```python
from build123d import *

# Parameters (mm, degrees)
SKETCH_1_W          = 120
SKETCH_1_H          = 19
EXTRUDE_1_DEPTH     = 3
SKETCH_2_R          = 1.5
CUT_EXTRUDE_1_DEPTH = 3


with BuildPart() as part:
    # Эскиз1 → Бобышка-Вытянуть1 (new body)
    with BuildSketch(Plane(origin=(0, 0, 0), x_dir=(1, 0, 0), z_dir=(0, 1, 0))):
        Rectangle(SKETCH_1_W, SKETCH_1_H)
    extrude(amount=EXTRUDE_1_DEPTH)

    # Эскиз2 → Вырез-Вытянуть1 (cut)
    with BuildSketch(Plane(origin=(0, 3, 0), x_dir=(1, 0, 0), z_dir=(0, 1, 0))):
        with Locations((-51.862444671, 3.5)):
            Circle(SKETCH_2_R)
        with Locations((-56.963668737, -3.5)):
            Circle(SKETCH_2_R)
        with Locations((-31.862444671, 3.5)):
            Circle(SKETCH_2_R)
        with Locations((-36.963668737, -3.5)):
            Circle(SKETCH_2_R)
        with Locations((-11.862444671, 3.5)):
            Circle(SKETCH_2_R)
        with Locations((-16.963668737, -3.5)):
            Circle(SKETCH_2_R)
        with Locations((8.137555329, 3.5)):
            Circle(SKETCH_2_R)
        with Locations((3.036331263, -3.5)):
            Circle(SKETCH_2_R)
        with Locations((28.137555329, 3.5)):
            Circle(SKETCH_2_R)
        with Locations((23.036331263, -3.5)):
            Circle(SKETCH_2_R)
        with Locations((48.137555329, 3.5)):
            Circle(SKETCH_2_R)
        with Locations((43.036331263, -3.5)):
            Circle(SKETCH_2_R)
    extrude(amount=-CUT_EXTRUDE_1_DEPTH, mode=Mode.SUBTRACT)


solid = part.part
```
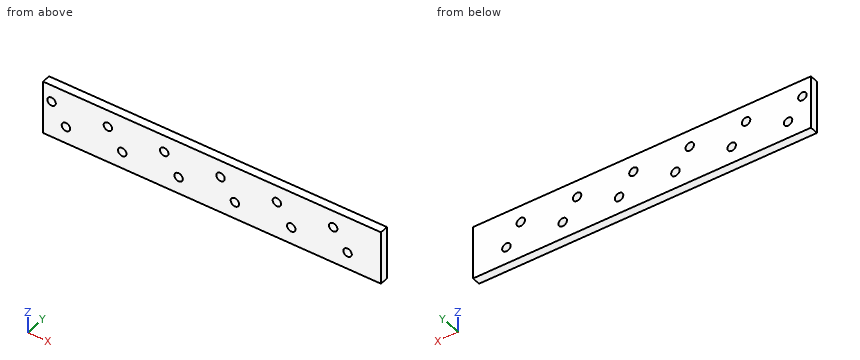
Source: CAD feature listing. Evaluate the final solid. Frame: model axes, mm. Coordinates: 2 decimals unless noted, no trailing zeros. Loops run counter-clockwise (first coordinate to the right, second up) from the corner with the lowest first, then second, coordinate; pieces in that order, holes last. Notation, with made-up numbers: M 6,23 L 61,23 A26 cw 61,49 Z; hole C 36.25,14 d7. An arc over 180 degrees is marked long. Put each result on its own line as item: value. Start each with the question number.
1) Cut plane C-C on x = -17. Return the cut outline in (y, z).
2) Contact query for flat-ended pins moving along their axis: pin 1 Ø2.5 at (x, z) = (-16.96, 3.5) entering from +Y; pin 2 Ø4 at (x, z) = (43.04, 3.5) entering from +Y. Output: stop coordinate, or through.
3) Cut plane B-B on y = 1.8. Give the number of separate pieces and of enclosed holes in the cut face, then the cut area to 3 significant figures.
4) Ray query, L1, parallel to Z at x = -11.5, y = 1.4; L2, parallel to Z at x = 4, y = 1. Return the intervals inside material, ascending. Write a range as from..to.
5) Cut plane A-A on z = 3.5. Return the cut outline in (x, y).
The answers:
1. outline: M 0,-9.5 L 3,-9.5 L 3,2 L 0,2 Z; M 0,5 L 3,5 L 3,9.5 L 0,9.5 Z
2. pin 1: passes through
2. pin 2: stops at y = 3
3. separate pieces: 1
3. enclosed holes: 12
3. area: 2,200 mm²
4. L1: z = -9.5..-4.96, -2.04..9.5
4. L2: z = -9.5..2.35, 4.65..9.5
5. outline: M -60,0 L -58.46,0 L -58.46,3 L -60,3 Z; M -55.46,0 L -38.46,0 L -38.46,3 L -55.46,3 Z; M -35.46,0 L -18.46,0 L -18.46,3 L -35.46,3 Z; M -15.46,0 L 1.54,0 L 1.54,3 L -15.46,3 Z; M 4.54,0 L 21.54,0 L 21.54,3 L 4.54,3 Z; M 24.54,0 L 41.54,0 L 41.54,3 L 24.54,3 Z; M 44.54,0 L 60,0 L 60,3 L 44.54,3 Z
